The drawing under review shows one solid part. Ordinate dimensions are in mm from its lowest x, y, z. A direction names the side the tool comes from. Round coordinates to 2 decimals unless told otherwise and drop trailing zeros. Order: outer loops, then holes, each group sorted by start corner. A loop starts at its lowest first (then second) coordinate and runs counter-clockwise, first axis right, second up. Notation, with made-up numbers: M 80,85.5 L 130,85.5 A26 cw 130,117.5 Z; hole C 69,63 d1. An arc over 180 degrees is marked long. Answer as a JSON object with one key per item and string values. Group by question number.
1. Machinability: for the marked faces 5 and 6, which of the approach directions +Z, -Z, +X, -X, +Y, -Y give a long, thin tool a straight path to every point of the face, cutting with its end or side? Answer none if there is none.
2. Mouldability with a two-part tool opening along X and no side actions: class the marked faces 1, 2, 3 and 4 as released by +X, released by -X, zero draft, split by the parting line, or undercut.
3. To check wall thickness, follow probe 1 along Z at (x, y) = (47.5, 314). State the ranges of the line that lie inside material, in increasing order. Write a range as [from, to].
4. Add section B-B on x = 49. State the section outline as (y, z) points.
5. Add section A-A on z = 33. State the section outline as (x, y) points.
6. Add section C-C on y = 332.5. State the section outline as (x, z) points.
7. Clearance check with a flat-ended pin moving along its axis: P1, Ø6, axis at x = 51.5, z = 9.5, coming from the -Y side. State where the tip first meets the part, or that it passes through.
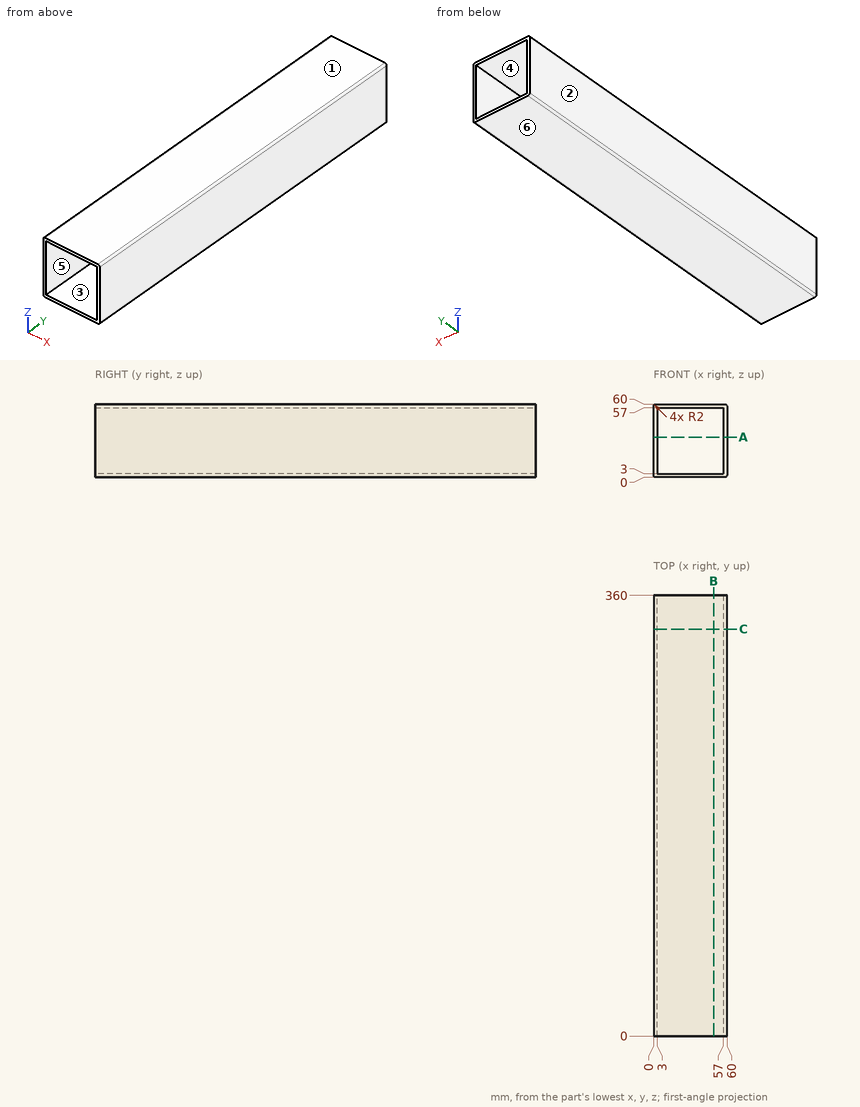
Recorded:
{
 "1": {"face 5": "+Y, -Y", "face 6": "-Z, +X, -X, +Y, -Y"},
 "2": {"face 1": "zero draft", "face 2": "released by -X", "face 3": "undercut", "face 4": "undercut"},
 "3": {"probe 1": "z = [0, 3], [57, 60]"},
 "4": {"outline": "M 0,0 L 360,0 L 360,3 L 0,3 Z; M 0,57 L 360,57 L 360,60 L 0,60 Z"},
 "5": {"outline": "M 0,0 L 3,0 L 3,360 L 0,360 Z; M 57,0 L 60,0 L 60,360 L 57,360 Z"},
 "6": {"outline": "M 0,2 A2 ccw 2,0 L 58,0 A2 ccw 60,2 L 60,58 A2 ccw 58,60 L 2,60 A2 ccw 0,58 Z; hole M 3,3 L 57,3 L 57,57 L 3,57 Z"},
 "7": {"P1": "passes through"}
}
